Work out the finished part from the listing and answer in its coordinate system (mm). Coordinates: 2 decimals unless noted, no trailing zeros. Loops run counter-clockwise (first coordinate to the right, second up) from the corner with the lowest first, then second, coordinate; pieces in that order, holes last. Notation, with made-up numbers: (26, 82) - (42, 82) arc R12 cw to (42, 90) - close; hole circle Ø6 at (28.5, 77). An arc over 180 degrees is marked (long way). Write each question's results on one line, items separated by ' | '. Start each with the question number.
1. Determine the mould class of faces 1 (the flat face through (0, 44.7, 0)), 2 (the cylindrical face through (-1.5, 21.35, -0.07)), 3 (the flat face through (1, 45, 1)) for opening direction X: released by +X, released by -X, zero draft, split by the parting line, or undercut.
2. Each of these flat-tipped pins is pushed along its axis until it touches: P1, Ø3, axis at x = -1.5, y = 29.5, coming from the -Z side; P2, Ø2, axis at y = 27, z = -1.5, coming from the -X side; P3, Ø1.5, axis at y = 21.5, z = -1, coming from the -X side. Where does it stop, or does it pass through?
3. Find the intervals of material crossed by line 1 along Y through (x, z) = (1.2, -0.05); line 2 along Z through (x, y) = (1.1, 23); line 3 along X through (y, z) = (20, 0.2), in increasing order. Write a range as [from, to].
4. A cutting plane is placed at A-A on y = 4. Determine the outline of the cut face in (x, z), then the cut area to 3 significant figures.
from build123d import *

# Parameters (mm, degrees)
SKETCH1_R           = 1.5
BOSS_EXTRUDE1_DEPTH = 45
SKETCH2_R           = 2.6
BOSS_EXTRUDE2_DEPTH = 1.7
BOSS_EXTRUDE2_TAPER = 32
SKETCH3_W           = 0.5
SKETCH3_H           = 1.758378485
SKETCH3_H_2         = 1.741621515
SKETCH3_W_2         = 1.734727157
SKETCH3_H_3         = 0.5
SKETCH3_W_3         = 1.765272843
CUT_EXTRUDE1_DEPTH  = 0.3


with BuildPart() as part:
    # Sketch1 → Boss-Extrude1 (new body)
    with BuildSketch(Plane(origin=(0, 0, 0), x_dir=(1, 0, 0), z_dir=(0, 1, 0))):
        Circle(SKETCH1_R)
    extrude(amount=BOSS_EXTRUDE1_DEPTH)

    # Sketch2 → Boss-Extrude2 (add)
    with BuildSketch(Plane(origin=(0, 45, 0), x_dir=(1, 0, 0), z_dir=(0, 1, 0))):
        Circle(SKETCH2_R)
    extrude(amount=-BOSS_EXTRUDE2_DEPTH, taper=BOSS_EXTRUDE2_TAPER)

    # Sketch3 → Cut-Extrude1 (cut)
    with BuildSketch(Plane(origin=(0, 45, 0), x_dir=(1, 0, 0), z_dir=(0, 1, 0))):
        with Locations((-0.015272843, 1.120810757)):
            Rectangle(SKETCH3_W, SKETCH3_H)
        with Locations((-0.015272843, -1.129189243)):
            Rectangle(SKETCH3_W, SKETCH3_H_2)
        with Locations((-1.132636421, -0.008378485)):
            Rectangle(SKETCH3_W_2, SKETCH3_H_3)
        with Locations((1.117363579, -0.008378485)):
            Rectangle(SKETCH3_W_3, SKETCH3_H_3)
        with Locations((-0.015272843, -0.008378485)):
            Rectangle(SKETCH3_W, SKETCH3_H_3)
    extrude(amount=-CUT_EXTRUDE1_DEPTH, mode=Mode.SUBTRACT)


solid = part.part
Values:
1) face 1: undercut | face 2: split by the parting line | face 3: zero draft
2) P1: z = -1.5 | P2: x = -1.41 | P3: x = -1.48
3) line 1: [0, 44.7] | line 2: [-1.02, 1.02] | line 3: [-1.49, 1.49]
4) outline: circle Ø3 at (0, 0) | area: 7.07 mm^2
